For this review, take the finished solid that the model builds, in its own axes (mm). A direction names the side the tool comes from. Coordinates: 2 decimals unless noted, no trailing zeros. Loops run counter-clockwise (first coordinate to the right, second up) from the corner with the lowest first, then second, coordinate; pieces in that order, holes last. Notation, with made-up numbers: (-22.75, 75.25) -> (13.25, 75.25) arc R19 ccw to (13.25, 110.25) -> close; hole circle Ø5 at (21, -17). An arc over 180 degrees is marked (long way). Use a Markdown table: item, result.
from build123d import *

# Parameters (mm, degrees)
F2_T     = -5.08
F5_DEPTH = 381
F6_W     = 183.9755326509
F6_H     = 374.7007958591
F7_DEPTH = 127


with BuildPart() as f1:
    # F0 (on Front) → F1 (revolve)
    with BuildSketch(Plane.XZ):
        with BuildLine():
            Line((0, 313.7035369873), (0, 0))
            Line((0, 0), (101.6, 0))
            Line((101.6, 0), (101.6, 72.2721558975))
            ThreePointArc((101.6, 72.2721558975), (151.9479695741, 197.5936266182), (82.9633497091, 313.7035369873))
            Line((82.9633497091, 313.7035369873), (0, 313.7035369873))
        make_face()
    revolve(axis=Axis((0, 0, 156.8517684937), (0, 0, -1)))

    # F2
    f2_openings = [f1.faces().sort_by_distance(p)[0] for p in [
        (0, 0, 0),
    ]]
    offset(amount=F2_T, openings=f2_openings, kind=Kind.INTERSECTION)

    # F4 (on offset) → F5 (cut)
    with BuildSketch(Plane.YZ.offset(177.8)):
        Polygon((-168.2938635349, -20.8534449339), (-40.0775820017, -20.8534449339), (-22.5597055078, -49.5606735349), (48.4589897096, -49.5606735349), (62.606588006, -20.8534449339), (175.8424788713, -20.8534449339), (175.8424788713, 336.9438350201), (0, 336.9438350201), (-10.2703914278, 381.5792500973), (-100.4313006997, 381.5792500973), (-107.4867025018, 336.9438350201), (-168.2938635349, 336.9438350201), align=None)
        Polygon((-10.2703914278, -20.8534449339), (-73.3597055078, 336.9438350201), (-22.5597055078, 336.9438350201), (40.5296085722, -20.8534449339), align=None, mode=Mode.SUBTRACT)
    extrude(amount=-F5_DEPTH, mode=Mode.SUBTRACT)

    # F6 (on Front) → F7 (cut, symmetric)
    with BuildSketch(Plane.XZ):
        with Locations((-91.9877663255, 152.6896301657)):
            Rectangle(F6_W, F6_H)
    extrude(amount=F7_DEPTH, both=True, mode=Mode.SUBTRACT)


solid = f1.part
(1) Take a section at D-D on z = 206. Write out the cut boundary in (x, y), plus the area to 3 significant figures.
Found:
| item | result |
|---|---|
| outline | (137.01, -50.27) -> (142.45, -50.27) arc R151.06 ccw to (151.06, 0.53) -> (145.94, 0.53) arc R145.94 cw to start |
| area | 266 mm^2 |
(2) Take a section at B-B on y = -3. Write out the cut boundary in (x, z), plus the area to 3 significant figures.
Found:
| item | result |
|---|---|
| outline | (96.47, 0) -> (101.56, 0) -> (101.56, 72.27) arc R152.37 ccw to (146.99, 226.02) -> (141.71, 226.02) arc R147.29 cw to (96.47, 74.57) -> close |
| area | 1,230 mm^2 |
(3) For line 1 along Z through (x, y) = (74, -30.5); line 2 along X through (y, z) = (1.5, 149); line 3 along Z through (x, y) = (103.5, -50.5), list the stretches that pass through material, from the lowest coordinate up.
Found:
| item | result |
|---|---|
| line 1 | z = 308.62 to 313.7 |
| line 2 | x = 142.63 to 147.87 |
| line 3 | z = 277.74 to 285.68 |
(4) Take a section at A-A on x = 107. Write out the cut boundary in (y, z), plus the area to 3 significant figures.
Found:
| item | result |
|---|---|
| outline | (-62.38, 274.67) -> (-60.98, 266.71) arc R101.26 cw to (-13.61, 286.21) -> (-14.87, 293.36) arc R108.52 ccw to start; (-29.65, 89.04) -> (-28.24, 81.08) arc R108.52 ccw to (22.79, 79.76) -> (21.53, 86.92) arc R101.26 cw to start |
| area | 750 mm^2 |
(5) For faces 1 (the face through (96.356, 5.628, 37.806)), 2 (the face through (97, 11, 0)), 3 (the face through (30, -43, 308.624)), 4 (the face through (31, -44, 313.704)), 5 (the face through (101.434, 5.802, 36.642)), list the 3-axis set-ups (+Z, -Z, +X, -X, +Y, -Y) from which the entire face can be reached by the end or side of a thin tool; tool diameter is ignored.
Found:
| item | result |
|---|---|
| face 1 | -Z, -X |
| face 2 | -Z, +X, -X, +Y, -Y |
| face 3 | -Z, -X, +Y |
| face 4 | +Z, +X, -X, +Y, -Y |
| face 5 | -Z, +X |
(6) Take a section at C-C on x = 25.5. Write out the cut boundary in (y, z).
Found:
| item | result |
|---|---|
| outline | (-69.26, 313.7) -> (-68.37, 308.62) -> (-17.57, 308.62) -> (-18.46, 313.7) -> close |
(7) For pin 1 Ø5 at (x, y) = (72, -56.5) entering from -Z; pin 2 Ø8 at (y, z) = (11.5, 189.5) entering from -X, all flat-tipped, find the tip position at first contact; note any pin that passes through.
Found:
| item | result |
|---|---|
| pin 1 | stops at z = 299.28 |
| pin 2 | passes through |
